Geometry check sheet. Reference: drawing and pictorial views, mm from the part's lowest x, y, z. Give positions to 0.01 mm unless a question says otherwise; leave off trailing zeros. Write each loop counter-clockwise with the first axis right and the second up, starting at its lowest first coordinate (ties: lowest second). Pieces come first, ordered by that corner, then holes. Notation, with made-up numbers: M 79.25,54 L 126.25,54 A16 ccw 126.25,85 Z; hole C 57.25,45.25 d9. An arc over 180 degrees is marked long. Write item = value, one per line. Start each with the question number.
1) Mould release check, pull along Z, two halves, no side actions. Record for the marked faces 1, 2, 3 and 4: released by +Z, released by -Z, zero draft, split by the parting line, or undercut.
2) Go/stop test with a flat-tipped pin: pin 1 (15 mm diameter, centred on x = 33.38, z = 37.58, fed in from +Y). Record where the tip stops, or that it passes through.
3) Cross-section at A-A, the plane x = 52. Record the cut outline in (y, z), plus the area to 3 significant figures.
4) Scan lines: line 1 along Z through (x, y) = (16.5, 18); line 2 along Z through (x, y) = (54, 38); line 3 along X through (y, z) = (2, 48.5) (1 decimal). Record each from-to range of solid material in increasing order. Write a range as [from, to].
5) Cross-section at C-C, the plane y = 24. Give the number of separate pieces and of enclosed holes in the cut face, plus the area to 3 significant figures.
6) Cross-section at B-B, the plane z = 36. Record the cut outline in (x, y) (1 decimal), plus the area to 3 significant figures.
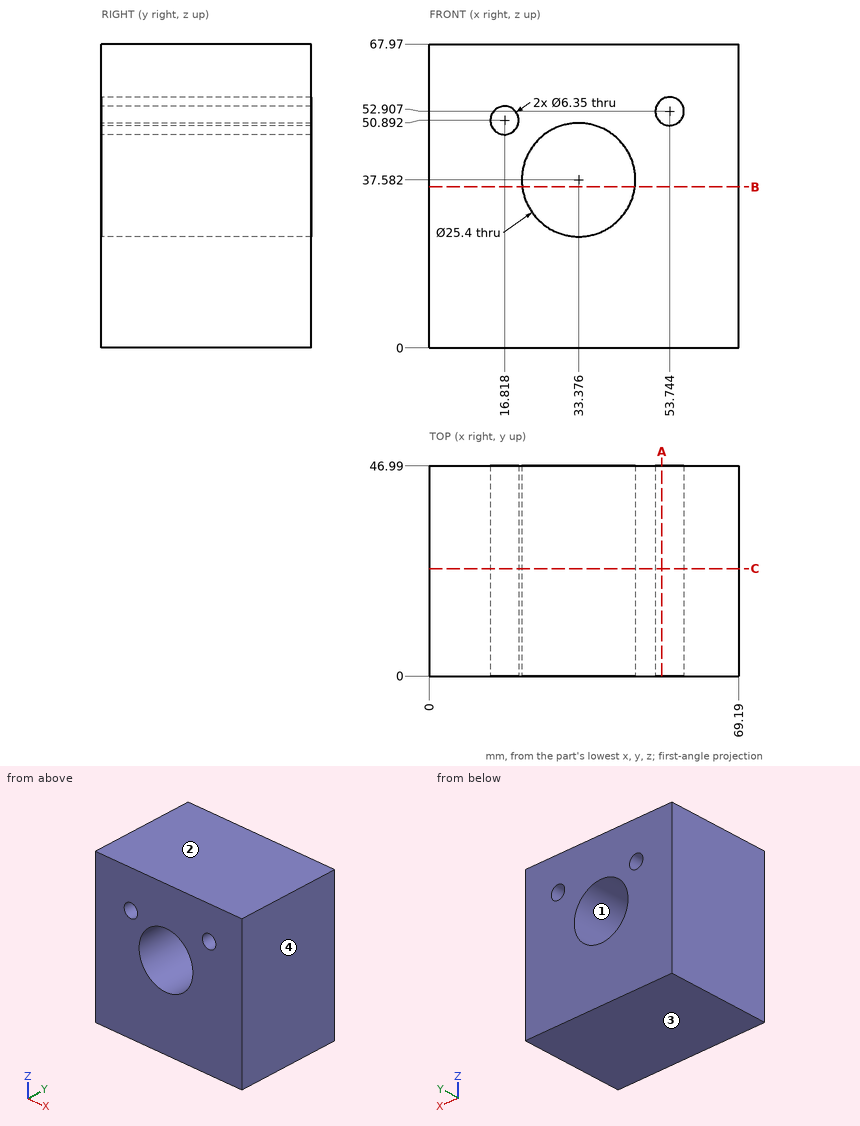
Reply:
q1.face_1 = undercut
q1.face_2 = released by +Z
q1.face_3 = released by -Z
q1.face_4 = zero draft
q2.pin_1 = through
q3.outline = M 0,0 L 46.99,0 L 46.99,50.25 L 0,50.25 Z; M 0,55.56 L 46.99,55.56 L 46.99,67.97 L 0,67.97 Z
q3.area = 2,940 mm2
q4.line_1 = [0, 47.73], [54.05, 67.97]
q4.line_2 = [0, 49.74], [56.07, 67.97]
q4.line_3 = [0, 14.7], [18.9, 26.9], [39.9, 69.2]
q5.separate_pieces = 1
q5.enclosed_holes = 3
q5.area = 4,130 mm2
q6.outline = M 0,0 L 20.8,0 L 20.8,47 L 0,47 Z; M 46,0 L 69.2,0 L 69.2,47 L 46,47 Z
q6.area = 2,070 mm2
